Build history of the part. All positions in model axes, mm. Face numbers are marked on the shaded views. A direction names the side the tool comes from. Round coordinates to 2 decimals unless told otherwise and drop trailing zeros. Loops run counter-clockwise (first coordinate to the right, second up) from the corner with the lowest first, then second, coordinate; pieces in that order, holes last. Notation, with made-up numbers: (84.25, 9.5) - (129.25, 9.5) arc R29 ccw to (129.25, 32.5) - close; hole circle Ø7 at (35.5, 44.5). An arc over 180 degrees is marked (long way). Use a Markdown table: item, result.
from build123d import *

# Parameters (mm, degrees)
SKETCH1_R           = 20
BOSS_EXTRUDE1_DEPTH = 3
SKETCH2_W           = 7
SKETCH2_H           = 36.693281072
BOSS_EXTRUDE2_DEPTH = 30
FILLET2_R           = 3
SKETCH3_R           = 21
SKETCH3_R_2         = 16
BOSS_EXTRUDE3_DEPTH = 7
SKETCH4_R           = 16
CUT_EXTRUDE1_DEPTH  = 7


with BuildPart() as part:
    # Sketch1 → Boss-Extrude1 (new body)
    with BuildSketch(Plane.XY):
        Circle(SKETCH1_R)
    extrude(amount=BOSS_EXTRUDE1_DEPTH)

    # Sketch2 → Boss-Extrude2 (add)
    with BuildSketch(Plane(origin=(0, 0, 0), x_dir=(-1, 0, 0), z_dir=(0, 0, -1))):
        Rectangle(SKETCH2_W, SKETCH2_H)
    extrude(amount=-BOSS_EXTRUDE2_DEPTH)

    # Fillet2
    fillet2_edges = [part.edges().sort_by_distance(p)[0] for p in [
        (3.5, 0, 3),
        (-3.5, 0, 3),
    ]]
    fillet(fillet2_edges, radius=FILLET2_R)

    # Sketch3 → Boss-Extrude3 (add)
    with BuildSketch(Plane.ZY.offset(3.5)):
        with Locations((34, 0)):
            Circle(SKETCH3_R)
        with Locations((34, 0)):
            Circle(SKETCH3_R_2, mode=Mode.SUBTRACT)
    extrude(amount=-BOSS_EXTRUDE3_DEPTH)

    # Sketch4 → Cut-Extrude1 (cut)
    with BuildSketch(Plane.ZY.offset(3.5)):
        with Locations(Location((34, 0, 0), (0, 0, 270))):
            Circle(SKETCH4_R)
    extrude(amount=-CUT_EXTRUDE1_DEPTH, mode=Mode.SUBTRACT)


solid = part.part
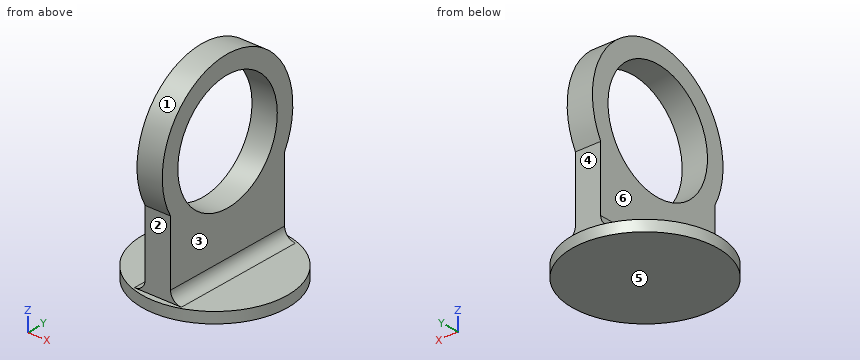
Q1. Cut at D-D, the plane y = 7.5. List the corners of the cut face in (x, z), plus the area to 3 significant figures.
Results found:
| item | result |
|---|---|
| outline | (-18.54, 0) - (18.54, 0) - (18.54, 3) - (6.5, 3) arc R3 cw to (3.5, 6) - (3.5, 19.87) - (-3.5, 19.87) - (-3.5, 6) arc R3 cw to (-6.5, 3) - (-18.54, 3) - close; (-3.5, 48.13) - (3.5, 48.13) - (3.5, 53.62) - (-3.5, 53.62) - close |
| area | 272 mm2 |
Q2. Cut at B-B, the plane z = 34. List the corners of the cut face in (x, y).
Results found:
| item | result |
|---|---|
| outline | (-3.5, -21) - (3.5, -21) - (3.5, -16) - (-3.5, -16) - close; (-3.5, 16) - (3.5, 16) - (3.5, 21) - (-3.5, 21) - close |
Q3. Pull direction Z, two halves, no side cores. Call the marked faces 4, 5 and 6: pulls with the +Z half, pulls with the -Z half, needs draft (parallel to the pull), parting line crosses it, or undercut.
Results found:
| item | result |
|---|---|
| face 4 | undercut |
| face 5 | pulls with the -Z half |
| face 6 | needs draft |
Q4. Which spindle directions (+Z, -Z, +X, -X, +Y, -Y) get a long thin tool onto all of the face, cutting with end or side? Do the marked faces 1, 2 and 3. Say none if no direction does.
Results found:
| item | result |
|---|---|
| face 1 | +X, -X |
| face 2 | +X, -X, -Y |
| face 3 | +Z, +X, +Y, -Y |
Q5. Cut at A-A, the plane y = 0. List the corners of the cut face in (x, z).
Results found:
| item | result |
|---|---|
| outline | (-20, 0) - (20, 0) - (20, 3) - (6.5, 3) arc R3 cw to (3.5, 6) - (3.5, 18) - (-3.5, 18) - (-3.5, 6) arc R3 cw to (-6.5, 3) - (-20, 3) - close; (-3.5, 50) - (3.5, 50) - (3.5, 55) - (-3.5, 55) - close |
Q6. Probe line 1 (Z direction, x = -1, y = 0); line 2 (Y direction, x = -1.25, z = 34); line 3 (X direction, y = -18, z = 31). List the from-to ranges inside material, lowest first.
Results found:
| item | result |
|---|---|
| line 1 | z = 0 to 18, 50 to 55 |
| line 2 | y = -21 to -16, 16 to 21 |
| line 3 | x = -3.5 to 3.5 |
Q7. Drop flat-ended pins along their axis: pin 1 (21 mm diameter, centred on y = -3, z = 24, fed in from -X); pin 2 (4 mm diameter, centred on y = -9.5, z = 23.5, fed in from +X); pin 3 (14.5 mm diameter, centred on x = 2, z = 9, fed in from +Y); pin 4 (6 mm diameter, centred on x = 7, z = 43, fed in from +Y). Give the stop position or say it passes through.
Results found:
| item | result |
|---|---|
| pin 1 | stops at x = -3.5 |
| pin 2 | stops at x = 3.5 |
| pin 3 | stops at y = 20 |
| pin 4 | passes through |
Q8. Cut at C-C, the plane x = 0. List the corners of the cut face in (y, z), plus the area to 3 significant figures.
Results found:
| item | result |
|---|---|
| outline | (-20, 0) - (20, 0) - (20, 3) - (18.35, 3) - (18.35, 23.78) arc R21 ccw (long way) to (-18.35, 23.78) - (-18.35, 3) - (-20, 3) - close; hole circle Ø32 at (0, 34) |
| area | 1,180 mm2 |
